from build123d import *

# Parameters (mm, degrees)
SKETCH1_W           = 60
SKETCH1_H           = 50
BOSS_EXTRUDE1_DEPTH = 10
SKETCH2_W           = 15
SKETCH2_H           = 30
CUT_REVOLVE1_ANGLE  = 120


with BuildPart() as part:
    # Sketch1 → Boss-Extrude1 (new, symmetric)
    with BuildSketch(Plane.XY):
        with Locations((0, 15)):
            Rectangle(SKETCH1_W, SKETCH1_H)
    extrude(amount=BOSS_EXTRUDE1_DEPTH, both=True)

    # Sketch2 → Cut-Revolve1 (revolve, cut)
    with BuildSketch(Plane.XY):
        with Locations((12.5, 15)):
            Rectangle(SKETCH2_W, SKETCH2_H)
    revolve(axis=Axis((0, 0, 0), (0, 1, 0)), revolution_arc=CUT_REVOLVE1_ANGLE, mode=Mode.SUBTRACT)


solid = part.part
Work out the finished part from the listing and answer in its coordinate system (mm). A direction names the side the tool comes from. Round coordinates to 2 decimals unless told otherwise and drop trailing zeros. Write each loop counter-clockwise with the first axis right and the second up, starting at its lowest first coordinate (ties: lowest second). Pieces come first, ordered by that corner, then holes. Notation, with made-up numbers: (-11.5, 52.25) - (42.5, 52.25) arc R12 ccw to (42.5, 75.25) - close; hole circle Ø6 at (71, 77). An arc over 180 degrees is marked (long way). Answer in a Markdown table with one row per item. Add a question column.
1. A cutting plane is placed at A-A, the plane x = 14.5. Determine the outline of the cut face in (y, z).
2. Find the intervals of material crossed by line 1 along Y through (x, z) = (-0.5, -5.25); line 2 along Z through (x, y) = (11.5, 8); line 3 along X through (y, z) = (13, -4), in increasing order. Write a range as from..to.
3. A cutting plane is placed at D-D, the plane z = -2.5. Determine the outline of the cut face in (x, y).
4. For faces 1 (the cylindrical face through (19.337, 15.21, -5.106)), 2 (the flat face through (-7, 15, -10)), 3 (the cylindrical face through (3, 15, -4)), determine the directions among +Z, -Z, +X, -X, +Y, -Y from which every point of the face is accessible in a straight line to the end or side of a thin tool.
5. The mould has two halves that part along Y. Classify faces 4 (the flat face through (30, 15, 0)), 5 (the flat face through (0, 40, 0)), 6 (the flat face through (10, 30, -5)): +Y half, -Y half, draft (parallel to the pull), parting line (faces both ways), or undercut.
6. A cutting plane is placed at C-C, the plane z = -6. Determine the outline of the cut face in (x, y), and give its area (3 significant figures).
7. A cutting plane is placed at B-B, the plane y = 24.5. Determine the outline of the cut face in (x, z), and give its area (3 significant figures).
Worked out:
| question | item | result |
|---|---|---|
| 1 | outline | (-10, -10) - (0, -10) - (0, 0) - (30, 0) - (30, -10) - (40, -10) - (40, 10) - (-10, 10) - close |
| 2 | line 1 | -10..0, 30..40 |
| 2 | line 2 | 0..10 |
| 2 | line 3 | -30..3, 19.6..30 |
| 3 | outline | (-30, -10) - (30, -10) - (30, 40) - (-30, 40) - close; hole (4.33, 0) - (19.84, 0) - (19.84, 30) - (4.33, 30) - close |
| 4 | face 1 | none |
| 4 | face 2 | -Z, +X, -X, +Y, -Y |
| 4 | face 3 | -Z |
| 5 | face 4 | draft |
| 5 | face 5 | +Y half |
| 5 | face 6 | undercut |
| 6 | outline | (-30, -10) - (30, -10) - (30, 40) - (-30, 40) - close; hole (-3.46, 0) - (19.08, 0) - (19.08, 30) - (-3.46, 30) - close |
| 6 | area | 2,320 mm^2 |
| 7 | outline | (-30, -10) - (-5.77, -10) - (-2.5, -4.33) arc R5 ccw to (5, 0) - (20, 0) arc R20 cw to (17.32, -10) - (30, -10) - (30, 10) - (-30, 10) - close |
| 7 | area | 1,010 mm^2 |
